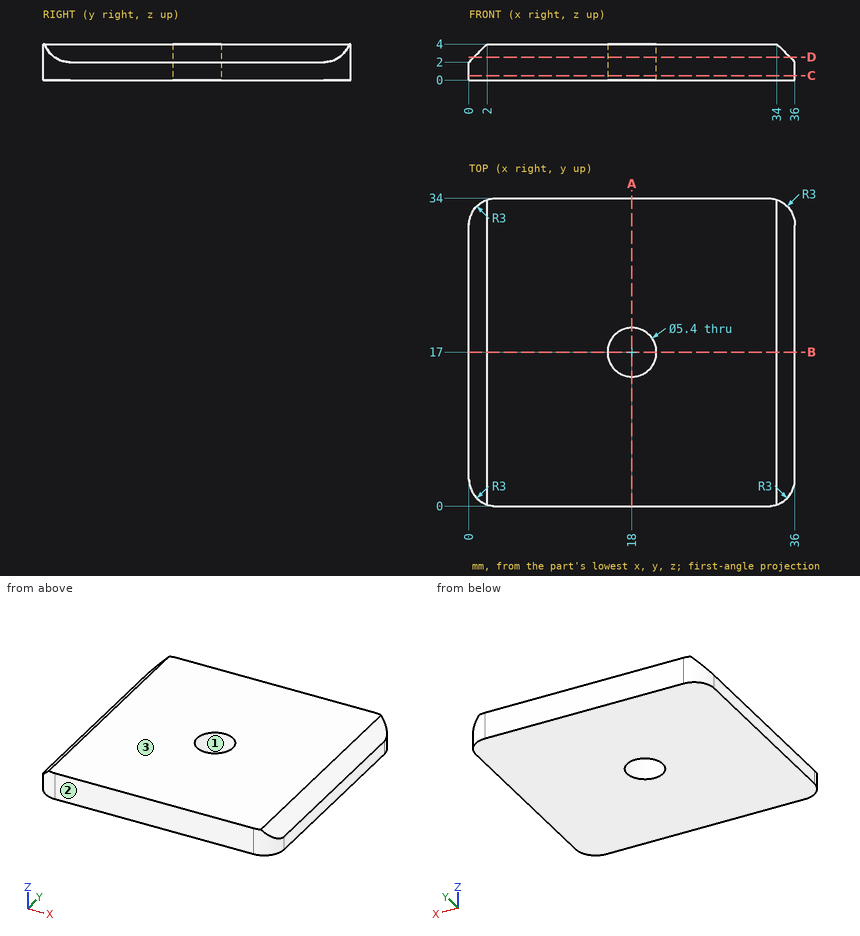
Drawing for the job (mm, zero at the part's lowest x, y, z). Round coordinates to 2 decimals unless told otherwise and drop trailing zeros. Write each loop counter-clockwise with the first axis right and the second up, starting at its lowest first coordinate (ties: lowest second). Pieces come first, ordered by that corner, then holes.
Item 1: Drill centre lines: L1, parallel to Y at x = 18, z = 1.55; L2, parallel to Y at x = 20, z = 0.85; L3, parallel to X at y = 12.5, z = 3.8. Where is each one in solid material? Low to high.
Filled in:
L1: y = 0 to 14.3, 19.7 to 34
L2: y = 0 to 15.19, 18.81 to 34
L3: x = 1.8 to 34.2
Item 2: Band-saw the part on A-A on x = 18. Write the cut outline in (y, z).
Filled in:
outline: (0, 0) - (14.3, 0) - (14.3, 4) - (0, 4) - close; (19.7, 0) - (34, 0) - (34, 4) - (19.7, 4) - close
Item 3: Band-saw the part on C-C on z = 0.5. Write the cut outline in (x, y).
Filled in:
outline: (0, 3) arc R3 ccw to (3, 0) - (33, 0) arc R3 ccw to (36, 3) - (36, 31) arc R3 ccw to (33, 34) - (3, 34) arc R3 ccw to (0, 31) - close; hole circle Ø5.4 at (18, 17)
Item 4: Band-saw the part on D-D on z = 2.55. Write the cut outline in (x, y), then the cut area to 3 significant figures.
Filled in:
outline: (0.55, 1.27) arc R3 ccw to (3, 0) - (33, 0) arc R3 ccw to (35.45, 1.27) - (35.45, 32.73) arc R3 ccw to (33, 34) - (3, 34) arc R3 ccw to (0.55, 32.73) - close; hole circle Ø5.4 at (18, 17)
area: 1,160 mm2
Item 5: Mould opens along Y. For the marked faces 1, 2 and 3 say: released by +Y, released by -Y, zero draft, split by the parting line, or undercut.
Filled in:
face 1: undercut
face 2: released by -Y
face 3: zero draft
Item 6: Band-saw the part on B-B on y = 17. Write the cut outline in (x, z), then the cut area to 3 significant figures.
Filled in:
outline: (0, 0) - (15.3, 0) - (15.3, 4) - (2, 4) - (0, 2) - close; (20.7, 0) - (36, 0) - (36, 2) - (34, 4) - (20.7, 4) - close
area: 118 mm2
Item 7: Drop a flat-ended pin along its axis: pin 1 Ø1.5 at (y, z) = (7.5, 3.5) entering from -X. Give the stop position or say it passes through.
Filled in:
pin 1: stops at x = 0.75
